from build123d import *

# Parameters (mm, degrees)
ESQUISSE1_R             = 11
BOSS_EXTRU_1_DEPTH      = 6.35
ENL_V_MAT_EXTRU_1_DEPTH = 135.686014493


with BuildPart() as part:
    # Esquisse1 → Boss.-Extru.1 (new body)
    with BuildSketch(Plane(origin=(0, 0, 0), x_dir=(1, 0, 0), z_dir=(0, 1, 0))):
        with BuildLine():
            Line((-96.654639651, 52.506938663), (-21.654639651, -77.493061337))
            ThreePointArc((-21.654639651, -77.493061337), (0, -90), (21.654639651, -77.493061337))
            Line((21.654639651, -77.493061337), (96.654639651, 52.506938663))
            ThreePointArc((96.654639651, 52.506938663), (96.648631983, 77.50346885), (75, 90))
            Line((75, 90), (-75, 90))
            ThreePointArc((-75, 90), (-96.648631983, 77.50346885), (-96.654639651, 52.506938663))
        make_face()
        with Locations(Location((0, 65, 0), (0, 0, 270))):
            Circle(ESQUISSE1_R, mode=Mode.SUBTRACT)
    extrude(amount=BOSS_EXTRU_1_DEPTH)

    # Esquisse3 → Enlèv. mat.-Extru.1 (cut, through all)
    with BuildSketch(Plane.XZ):
        Polygon((-79.572614132, -82), (-77.286307066, -85.96), (-72.713692934, -85.96), (-70.427385868, -82), (-72.713692934, -78.04), (-77.286307066, -78.04), align=None)
        Polygon((-94.295045996, -56.5), (-92.00873893, -60.46), (-87.436124798, -60.46), (-85.149817732, -56.5), (-87.436124798, -52.54), (-92.00873893, -52.54), align=None)
        Polygon((-64.850182268, -56.5), (-62.563875202, -60.46), (-57.99126107, -60.46), (-55.704954004, -56.5), (-57.99126107, -52.54), (-62.563875202, -52.54), align=None)
        Polygon((55.704954004, -56.5), (57.99126107, -60.46), (62.563875202, -60.46), (64.850182268, -56.5), (62.563875202, -52.54), (57.99126107, -52.54), align=None)
        Polygon((70.427385868, -82), (72.713692934, -85.96), (77.286307066, -85.96), (79.572614132, -82), (77.286307066, -78.04), (72.713692934, -78.04), align=None)
        Polygon((85.149817732, -56.5), (87.436124798, -60.46), (92.00873893, -60.46), (94.295045996, -56.5), (92.00873893, -52.54), (87.436124798, -52.54), align=None)
        Polygon((-4.572614132, 48), (-2.286307066, 44.04), (2.286307066, 44.04), (4.572614132, 48), (2.286307066, 51.96), (-2.286307066, 51.96), align=None)
        Polygon((-19.295045996, 73.5), (-17.00873893, 69.54), (-12.436124798, 69.54), (-10.149817732, 73.5), (-12.436124798, 77.46), (-17.00873893, 77.46), align=None)
        Polygon((10.149817732, 73.5), (12.436124798, 69.54), (17.00873893, 69.54), (19.295045996, 73.5), (17.00873893, 77.46), (12.436124798, 77.46), align=None)
    extrude(amount=-ENL_V_MAT_EXTRU_1_DEPTH, mode=Mode.SUBTRACT)


solid = part.part
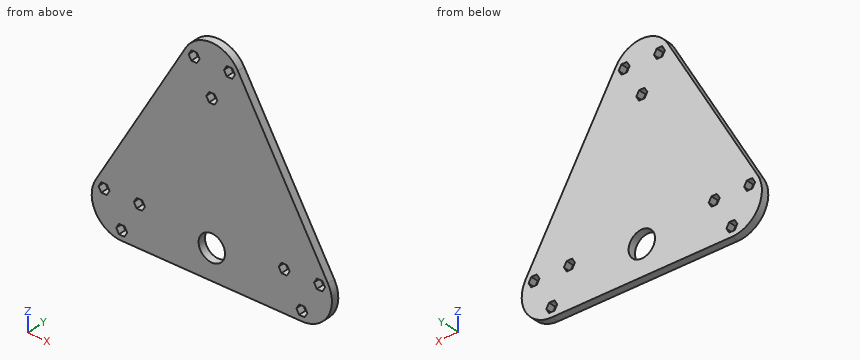
For this review, take the finished solid that the model builds, in its own axes (mm). Coordinates: 2 decimals unless noted, no trailing zeros. Order: outer loops, then holes, each group sorted by start corner. A loop starts at its lowest first (then second) coordinate and runs counter-clockwise, first axis right, second up. Notation, with made-up numbers: (-3, 2) -> (56, 2) arc R15 cw to (56, 7) -> close; hole circle Ø2 at (2.5, 23.25). An arc over 180 degrees is marked (long way). Return JSON: item names as keys, results as strings.
1. We need section A-A on z = -65. Write out the cut boundary in (x, y), and give its area (3 significant figures).
Answer block:
{"outline": "(-100, 0) -> (-11, 0) -> (-11, 6.35) -> (-100, 6.35) -> close; (11, 0) -> (100, 0) -> (100, 6.35) -> (11, 6.35) -> close", "area": "1,130 mm²"}
2. We need section B-B on x = 0. Write out the cut boundary in (y, z).
Answer block:
{"outline": "(0, -90) -> (6.35, -90) -> (6.35, -76) -> (0, -76) -> close; (0, -54) -> (6.35, -54) -> (6.35, 44.04) -> (0, 44.04) -> close; (0, 51.96) -> (6.35, 51.96) -> (6.35, 90) -> (0, 90) -> close"}
3. For line 1 (X direction, y = 2, z = -65); line 2 (X direction, y = 1, z = -11); line 3 (X direction, y = 3, z = 45), list the stretches that pass through material, from the lowest coordinate up. Write a range as from..to.
Answer block:
{"line 1": "-100..-11, 11..100", "line 2": "-72.71..72.71", "line 3": "-40.4..-2.84, 2.84..40.4"}
4. For pin 1 Ø3.5 at (x, y) = (59.5, 3.5) entering from +Z; pin 2 Ø2.5 at (x, y) = (-90.5, 2.5) entering from -Z; pin 3 Ø3.5 at (x, y) = (90, 4.5) entering from -Z, all flat-tipped, find the tip position at first contact; note any pin that passes through.
Answer block:
{"pin 1": "z = 14.93", "pin 2": "z = -85.54", "pin 3": "z = -86.2"}
5. We need section C-C on y = 2.5. State how many separate pieces and enclosed holes the cut face has, and give its area (3 significant figures).
Answer block:
{"separate pieces": "1", "enclosed holes": "10", "area": "22,100 mm²"}
6. We need section D-D on z = -17. Write out the cut boundary in (x, y).
Answer block:
{"outline": "(-76.17, 0) -> (76.17, 0) -> (76.17, 6.35) -> (-76.17, 6.35) -> close"}
